Input: part model. Units: mm. Frame: model coordinates. Face numbers are marked on the shaded views. A direction names the side the tool comes from. Coordinates: 2 decimals unless noted, no trailing zeros. Order: outer loops, then holes, each group sorted by start corner. A loop starts at its lowest first (then second) coordinate and runs counter-clockwise, first axis right, second up. Notation, with made-up numbers: (52.25, -16.5) -> (82.25, -16.5) arc R22 cw to (82.25, -8.5) -> close; hole circle Ø3 at (-15.5, 68.5). An arc over 180 degrees is marked (long way). One line per question, with ' | ' between items.
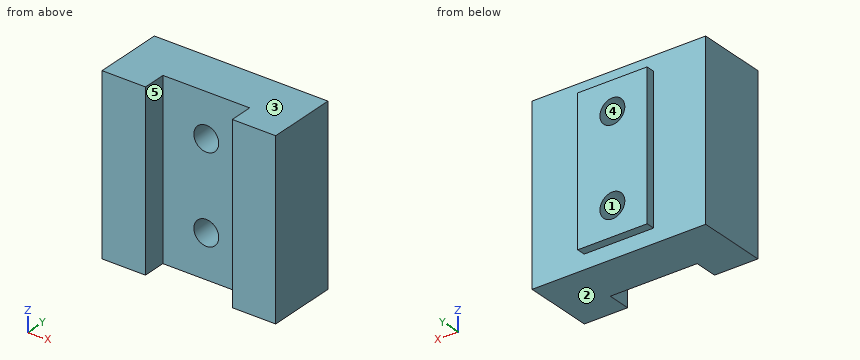
```python
from build123d import *

# Parameters (mm, degrees)
SKETCH1_W           = 30
SKETCH1_H           = 30
BOSS_EXTRUDE1_DEPTH = 12
SKETCH2_R           = 2.15
CUT_EXTRUDE1_DEPTH  = 25.372115214
BOSS_EXTRUDE2_START = 1.5
SKETCH2_3_W         = 12
SKETCH2_3_H         = 25
SKETCH2_3_R         = 2.15
BOSS_EXTRUDE2_DEPTH = 1.5
SKETCH3_W           = 15
SKETCH3_H           = 30
CUT_EXTRUDE2_DEPTH  = 4


with BuildPart() as part:
    # Sketch1 → Boss-Extrude1 (new body)
    with BuildSketch(Plane(origin=(0, 0, 0), x_dir=(1, 0, 0), z_dir=(0, 1, 0))):
        Rectangle(SKETCH1_W, SKETCH1_H)
    extrude(amount=BOSS_EXTRUDE1_DEPTH)

    # Sketch2 → Cut-Extrude1 (cut, through all)
    with BuildSketch(Plane(origin=(0, 12, 0), x_dir=(1, 0, 0), z_dir=(0, 1, 0))):
        with Locations(Location((0, -7.5, 0), (0, 0, 270))):
            Circle(SKETCH2_R)
        with Locations(Location((0, 7.5, 0), (0, 0, 270))):
            Circle(SKETCH2_R)
    extrude(amount=-CUT_EXTRUDE1_DEPTH, mode=Mode.SUBTRACT)

    # Sketch2_3 → Boss-Extrude2 (add)
    with BuildSketch(Plane(origin=(0, 12, 0), x_dir=(1, 0, 0), z_dir=(0, 1, 0)).offset(BOSS_EXTRUDE2_START)):
        Rectangle(SKETCH2_3_W, SKETCH2_3_H)
        with Locations(Location((0, -7.5, 0), (0, 0, 270))):
            Circle(SKETCH2_3_R, mode=Mode.SUBTRACT)
        with Locations(Location((0, 7.5, 0), (0, 0, 270))):
            Circle(SKETCH2_3_R, mode=Mode.SUBTRACT)
    extrude(amount=-BOSS_EXTRUDE2_DEPTH)

    # Sketch3 → Cut-Extrude2 (cut)
    with BuildSketch(Plane.XZ):
        Rectangle(SKETCH3_W, SKETCH3_H)
    extrude(amount=-CUT_EXTRUDE2_DEPTH, mode=Mode.SUBTRACT)


solid = part.part
```
1. Pin query (flat end, axial travel): pin 1 Ø10 at (x, z) = (1, -3) entering from -Y. Return the tip coordinate at first contact, or that it passes through.
Recorded:
pin 1: stops at y = 4
2. Cut plane B-B, the plane x = 0. Return loops of the section in (y, z).
Recorded:
outline: (4, -15) -> (12, -15) -> (12, -12.5) -> (13.5, -12.5) -> (13.5, -9.65) -> (4, -9.65) -> close; (4, -5.35) -> (13.5, -5.35) -> (13.5, 5.35) -> (4, 5.35) -> close; (4, 9.65) -> (13.5, 9.65) -> (13.5, 12.5) -> (12, 12.5) -> (12, 15) -> (4, 15) -> close
3. Cut plane C-C, the plane y = 3.5. Return loops of the section in (x, z).
Recorded:
outline: (-15, -15) -> (-7.5, -15) -> (-7.5, 15) -> (-15, 15) -> close; (7.5, -15) -> (15, -15) -> (15, 15) -> (7.5, 15) -> close
4. Mould query, pull axis Z, two halves, no side actions, for the marked faces 1, 2 and 3. Classes: released by +Z, released by -Z, zero draft, split by the parting line, or undercut.
Recorded:
face 1: undercut | face 2: released by -Z | face 3: released by +Z
5. Cut plane D-D, the plane z = 1.5. Return loops of the section in (x, y).
Recorded:
outline: (-15, 0) -> (-7.5, 0) -> (-7.5, 4) -> (7.5, 4) -> (7.5, 0) -> (15, 0) -> (15, 12) -> (6, 12) -> (6, 13.5) -> (-6, 13.5) -> (-6, 12) -> (-15, 12) -> close
6. Ray query, line 1 (X direction, y = 8.25, z = -7.5); line 2 (X direction, y = 2.5, z = -7); line 3 (Y direction, x = -11.25, z = 12). Return the intervals inside material, ascending. Write a range as [from, to].
Recorded:
line 1: x = [-15, -2.15], [2.15, 15] | line 2: x = [-15, -7.5], [7.5, 15] | line 3: y = [0, 12]
7. Cut plane A-A, the plane z = -7.5. Return loops of the section in (x, y).
Recorded:
outline: (-15, 0) -> (-7.5, 0) -> (-7.5, 4) -> (-2.15, 4) -> (-2.15, 13.5) -> (-6, 13.5) -> (-6, 12) -> (-15, 12) -> close; (2.15, 4) -> (7.5, 4) -> (7.5, 0) -> (15, 0) -> (15, 12) -> (6, 12) -> (6, 13.5) -> (2.15, 13.5) -> close
8. Access query for the marked faces 4 and 5. Directions: +Z, -Z, +X, -X, +Y, -Y. A direction counts if a zero-diameter tool reaches every point of the face in a straight line with its end or side. Return the directions, or none.
Recorded:
face 4: +Y, -Y | face 5: +Z, -Z, -Y
